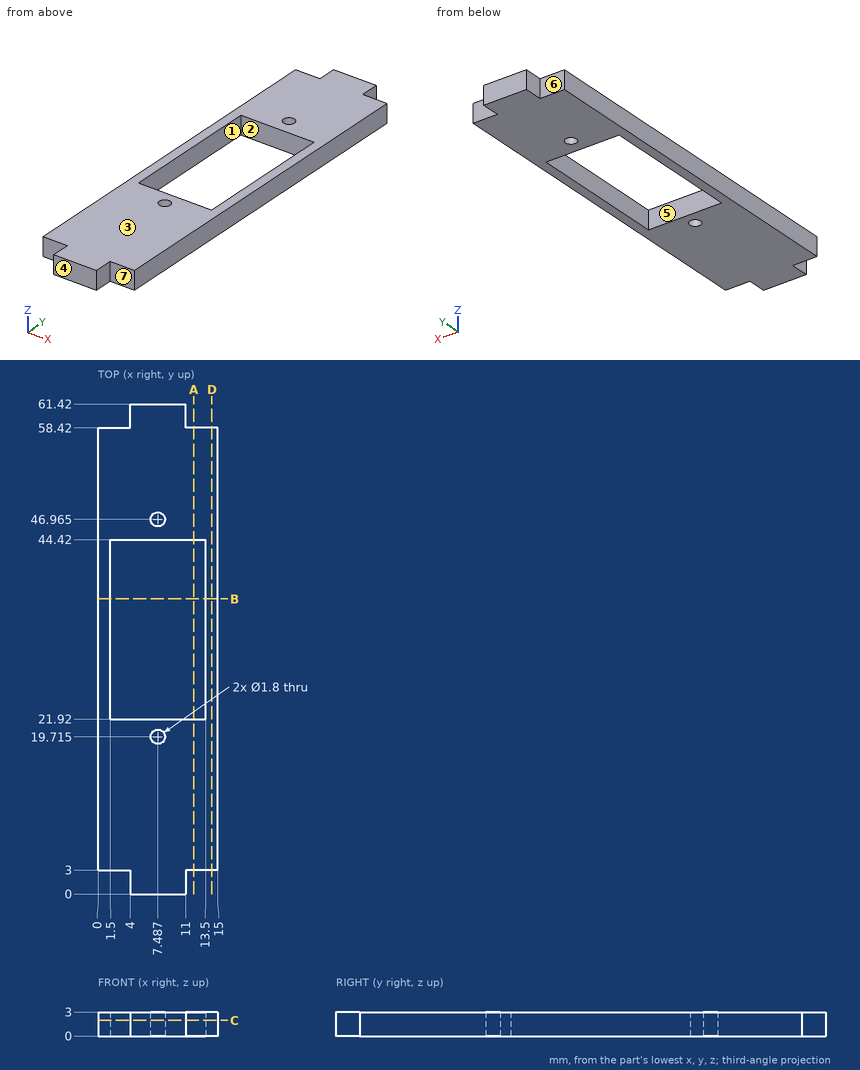
Source: three-view drawing plus pictorial views. Frame: mm from the lowest corner of the part. A direction names the side the tool comes from. Coordinates: 2 decimals unless noted, no trailing zeros. Order: outer loops, then holes, each group sorted by start corner. A loop starts at its lowest first (then second) coordinate and runs counter-clockwise, first axis right, second up.
1) Section B-B (y = 37). Return loops of the section in (x, z).
Result sheet:
outline: (0, 0) - (1.5, 0) - (1.5, 3) - (0, 3) - close; (13.5, 0) - (15, 0) - (15, 3) - (13.5, 3) - close
2) Set-up query: the marked faces 5, 6 and 7. Return all of +Z, -Z, +X, -X, +Y, -Y with unobstructed straight access to the full face (end or side cutting, diameter ignored); none if empty.
Result sheet:
face 5: +Z, -Z
face 6: +Z, -Z, -X, +Y
face 7: +Z, -Z, +X, -Y
3) Ray query, probe 1 along Y at (x, z) = (7.5, 2.9) (3 decimals); probe 2 along Y at (x, z) = (7.25, 0.4); probe 3 along X at (y, z) = (23, 2.6). Return the intervals inside material, ascending.
Result sheet:
probe 1: y = 0 to 18.815, 20.615 to 21.92, 44.42 to 46.065, 47.865 to 61.42
probe 2: y = 0 to 18.85, 20.58 to 21.92, 44.42 to 46.1, 47.83 to 61.42
probe 3: x = 0 to 1.5, 13.5 to 15
4) Draft query along Y for the marked faces 1, 2, 3 and 4. Return one class per face: released by +Y, released by -Y, zero draft, split by the parting line, or undercut.
Result sheet:
face 1: undercut
face 2: undercut
face 3: zero draft
face 4: released by -Y
5) Section C-C (z = 1.95). Return loops of the section in (x, y) (3 decimals).
Result sheet:
outline: (0, 3) - (4, 3) - (4, 0) - (11, 0) - (11, 3) - (15, 3) - (15, 58.42) - (11, 58.42) - (11, 61.42) - (4, 61.42) - (4, 58.42) - (0, 58.42) - close; hole (1.5, 21.92) - (13.5, 21.92) - (13.5, 44.42) - (1.5, 44.42) - close; hole circle Ø1.8 at (7.487, 19.715); hole circle Ø1.8 at (7.487, 46.965)
6) First-contact query: P1, Ø1.5, axis at x = 3, z = 1.5, coming from the -Y side; P2, Ø0.9, axis at y = 60.5, z = 2, coming from the +X side; P3, Ø1.5, axis at x = 13.5, z = 1.5, coming from the +Y side. Flat tips, straight axial feed; report the tip coordinate or a pass-through.
Result sheet:
P1: stops at y = 3
P2: stops at x = 11
P3: stops at y = 58.42
7) Section D-D (x = 14.25). Return loops of the section in (y, z).
Result sheet:
outline: (3, 0) - (58.42, 0) - (58.42, 3) - (3, 3) - close
8) Section A-A (x = 12). Return loops of the section in (y, z).
Result sheet:
outline: (3, 0) - (21.92, 0) - (21.92, 3) - (3, 3) - close; (44.42, 0) - (58.42, 0) - (58.42, 3) - (44.42, 3) - close
